Geometry check sheet. Reference: drawing and pictorial views, mm from the part's lowest x, y, z. Coordinates: 2 decimals unless noted, no trailing zeros. Order: outer loops, then holes, each group sorted by start corner. A loop starts at its lowest first (then second) coordinate and runs counter-clockwise, first axis right, second up. Notation, with made-up numbers: (35, -16.5) -> (72, -16.5) arc R22 cw to (72, 21.5) -> close; hole circle Ø1 at (5, 71.25). An arc over 180 degrees is marked (long way). Use CSV: the item, a comma, the result in double quotes. Start each with the question number.
1) Scan lines: line 1 along Y through (x, z) = (6.5, 0.25) (3 decimals); line 2 along X through (y, z) = (14, 0.7) (3 decimals); line 3 along Y through (x, z) = (22.5, 0.7). Record each from-to range of solid material in increasing order.
2) Sectioned sample at B-B on x = 12. Record the boundary of the cut face in (y, z) (3 decimals).
3) Sectioned sample at C-C on z = 3.55. Record the boundary of the cut face in (x, y) (1 decimal).
4) Sectioned sample at A-A on y = 42. Record the boundary of the cut face in (x, z) (3 decimals), then the cut area to 3 significant figures.
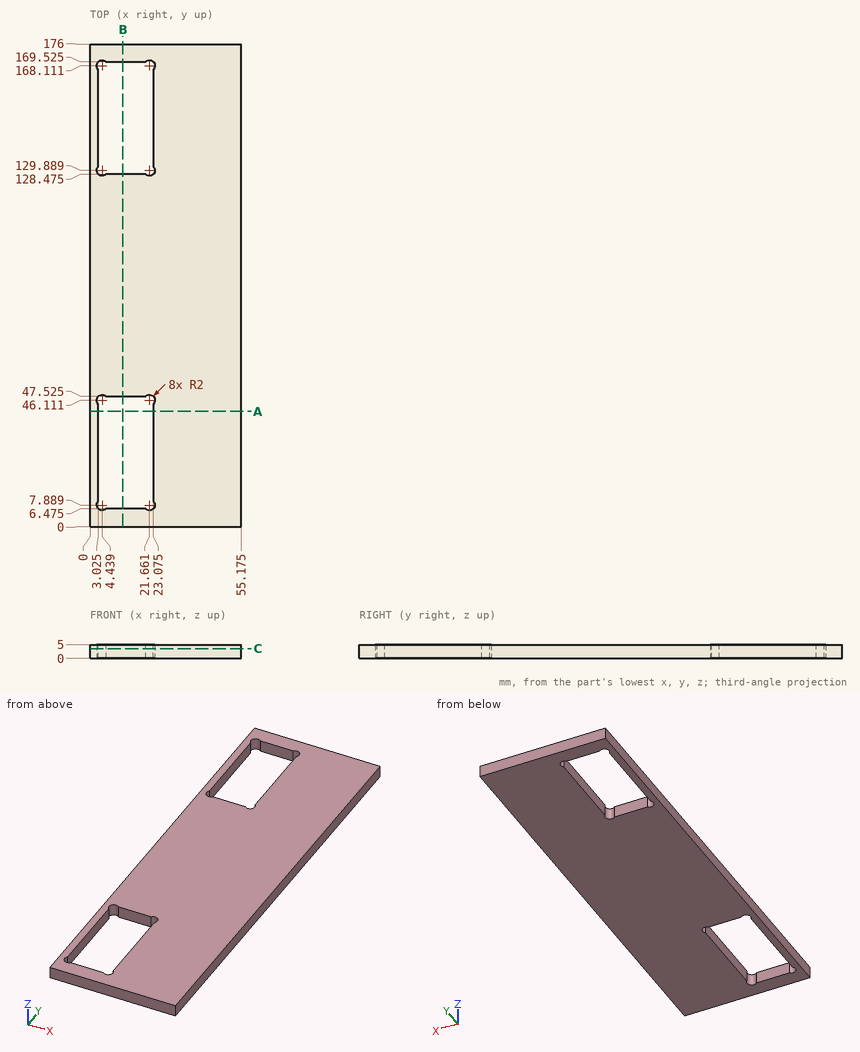
Answers follow:
1,line 1,"y = 0 to 6.475, 47.525 to 128.475, 169.525 to 176"
1,line 2,"x = 0 to 3.025, 23.075 to 55.175"
1,line 3,"y = 0 to 6.07, 47.93 to 128.07, 169.93 to 176"
2,outline,"(0, 0) -> (6.475, 0) -> (6.475, 5) -> (0, 5) -> close; (47.525, 0) -> (128.475, 0) -> (128.475, 5) -> (47.525, 5) -> close; (169.525, 0) -> (176, 0) -> (176, 5) -> (169.525, 5) -> close"
3,outline,"(0, 0) -> (55.2, 0) -> (55.2, 176) -> (0, 176) -> close; hole (3, 9.3) arc R2 ccw to (5.9, 6.5) -> (20.2, 6.5) arc R2 ccw to (23.1, 9.3) -> (23.1, 44.7) arc R2 ccw to (20.2, 47.5) -> (5.9, 47.5) arc R2 ccw to (3, 44.7) -> close; hole (3, 131.3) arc R2 ccw to (5.9, 128.5) -> (20.2, 128.5) arc R2 ccw to (23.1, 131.3) -> (23.1, 166.7) arc R2 ccw to (20.2, 169.5) -> (5.9, 169.5) arc R2 ccw to (3, 166.7) -> close"
4,outline,"(0, 0) -> (3.025, 0) -> (3.025, 5) -> (0, 5) -> close; (23.075, 0) -> (55.175, 0) -> (55.175, 5) -> (23.075, 5) -> close"
4,area,"176 mm²"
